For this review, take the finished solid that the model builds, in its own axes (mm). A direction names the side the tool comes from. Give positions to 0.01 mm unless a question says otherwise; leave off trailing zeros. Write each loop counter-clockwise with the first axis right and the second up, starting at its lowest first coordinate (ties: lowest second). Pieces come first, ordered by that corner, then holes.
1) We need section D-D on x = -26. Give the boundary of the cut face in (y, z), and give its area (3 significant figures).
2) We need section A-A on y = -9. Give the number of separate pieces and of enclosed holes in the cut face, and give its area (3 significant figures).
3) We need section B-B on y = 11. Give the boundary of the cut face in (x, z).
4) Machinability: for faces 4 (the face through (-11.5, 15, 3)), 5 (the face through (-15, -9, 1)), 6 (the face through (21.95, -3.8, 3.52)), which of the approach directions +Z, -Z, +X, -X, +Y, -Y give a long, thin tool a straight path to every point of the face, cutting with its end or side? Answer none if there is none.
5) Wall thickness on line 1 along Y through (x, z) = (-1, 1.5); line 2 along Y through (x, z) = (-25, 1.2); line 3 along X through (y, z) = (26, 0.8): over which ranges is each line inside the solid? List them lowest first.
6) For P1, Ø3, axis at x = 21, y = -10, coming from the +Z side; P2, Ø1.5, axis at y = 12, z = 3.5, coming from the -X side; P3, Ø0.9, axis at y = 13, z = 4, coming from the +X side, all flat-tipped, find the tip position at first contact; note any pin that passes through.
7) Draft analysis for pull direction Y (two halves, no side actions). For faces 1 (the face through (0, 7.15, 3)), 2 (the face through (28.5, -31.07, 1.01)), 3 (the face through (0, 6, 5)), state which applies: pulls with the +Y half, pulls with the -Y half, needs draft (parallel to the pull), parting line crosses it, or undercut.
from build123d import *

# Parameters (mm, degrees)
F0_W      = 60
F0_H      = 65
F1_DEPTH  = 2
F2_W      = 20
F2_H      = 12.7
F3_DEPTH  = 25
F4_R      = 1.75
F4_W      = 30
F4_H      = 22
F5_DEPTH  = 25
F7_DEPTH  = 3
F8_SIZE   = 2.99999
F10_D     = 4.5
F11_R     = 5
F12_W     = 48
F12_H     = 19.7
F12_W_2   = 23
F12_H_2   = 15.7
F13_DEPTH = 3
F14_SIZE  = 5


# Not quite as in the source:
# - a fillet or chamfer is up to 0.001 mm smaller than in the source, because OpenCascade refuses the exact size
# - a pattern or mirror of a feature is missing from the dataset's text; its kind, count and spacing are read off the source's solid


with BuildPart() as f1:
    # F0 (on Top) → F1 (new body)
    with BuildSketch(Plane.XY):
        Rectangle(F0_W, F0_H)
    extrude(amount=F1_DEPTH)

    # F2 (on face) → F3 (cut)
    with BuildSketch(Plane.XY.offset(2)):
        with Locations((0, 15)):
            Rectangle(F2_W, F2_H)
    extrude(amount=-F3_DEPTH, mode=Mode.SUBTRACT)

    # F4 (on face) → F5 (cut)
    with BuildSketch(Plane.XY.offset(2)):
        with Locations((-20, -9)):
            Circle(F4_R)
        with Locations((0, -9)):
            Rectangle(F4_W, F4_H)
        with Locations((20, -9)):
            Circle(F4_R)
    extrude(amount=-F5_DEPTH, mode=Mode.SUBTRACT)

    # F6 (on face) → F7 (join)
    with BuildSketch(Plane.XY.offset(2)):
        Polygon((-24, -6.6905989232), (-24, -11.3094010768), (-20, -13.6188021535), (-16, -11.3094010768), (-16, -6.6905989232), (-20, -4.3811978465), align=None)
        Polygon((-20, -12.3486315613), (-22.9, -10.6743157806), (-22.9, -7.3256842194), (-20, -5.6513684387), (-17.1, -7.3256842194), (-17.1, -10.6743157806), align=None, mode=Mode.SUBTRACT)
    f7 = extrude(amount=F7_DEPTH)

    # F7_copies: F7 across plane
    add(f7.mirror(Plane(origin=(0, 0, 0), x_dir=(0, 0, 1), z_dir=(1, 0, 0))))

    # F8 (size 3 in the source; OpenCascade refuses exactly that, so slightly less here)
    f8_edges = [f1.edges().sort_by_distance(p)[0] for p in [
        (-22, -12.464102, 2),
        (-18, -12.464102, 2),
        (-22, -5.535898, 2),
        (-18, -5.535898, 2),
        (18, -5.535898, 2),
        (18, -12.464102, 2),
        (22, -12.464102, 2),
        (22, -5.535898, 2),
    ]]
    chamfer(f8_edges, length=F8_SIZE)

    # F10 (through all)
    with Locations(Plane.XY.offset(2)):
        with Locations((-25, 27.5), (25, 27.5), (25, -27.5), (-25, -27.5)):
            Hole(F10_D / 2)

    # F11
    f11_edges = [f1.edges().sort_by_distance(p)[0] for p in [
        (30, 32.5, 1),
        (-30, 32.5, 1),
        (30, -32.5, 1),
        (-30, -32.5, 1),
    ]]
    fillet(f11_edges, radius=F11_R)

    # F12 (on face) → F13 (join)
    with BuildSketch(Plane.XY.offset(2)):
        with Locations((0, 15)):
            Rectangle(F12_W, F12_H)
        with Locations((0, 15)):
            Rectangle(F12_W_2, F12_H_2, mode=Mode.SUBTRACT)
    extrude(amount=F13_DEPTH)

    # F14
    f14_edges = [f1.edges().sort_by_distance(p)[0] for p in [
        (24, 24.85, 3.5),
        (-24, 24.85, 3.5),
    ]]
    chamfer(f14_edges, length=F14_SIZE)


solid = f1.part
Results list:
1. outline: (-32.4, 0) - (-29.52, 0) - (-29.52, 2) - (-32.4, 2) - close; (-25.48, 0) - (25.48, 0) - (25.48, 2) - (-25.48, 2) - close; (29.52, 0) - (32.4, 0) - (32.4, 2) - (29.52, 2) - close
1. area: 113 mm2
2. separate pieces: 4
2. enclosed holes: 0
2. area: 59.2 mm2
3. outline: (-30, 0) - (-10, 0) - (-10, 2) - (-11.5, 2) - (-11.5, 5) - (-24, 5) - (-24, 2) - (-30, 2) - close; (10, 0) - (30, 0) - (30, 2) - (24, 2) - (24, 5) - (11.5, 5) - (11.5, 2) - (10, 2) - close
4. face 4: +Z
4. face 5: +Z, -Z
4. face 6: +Z, +X
5. line 1: y = -32.5 to -20, 2 to 8.65, 21.35 to 32.5
5. line 2: y = -32.5 to -29.75, -25.25 to 25.25, 29.75 to 32.5
5. line 3: x = -30 to -26.68, -23.32 to 23.32, 26.68 to 30
6. P1: stops at z = 2
6. P2: stops at x = -24
6. P3: stops at x = 24
7. face 1: undercut
7. face 2: pulls with the -Y half
7. face 3: needs draft
